Can you work these out from the model? Positions are in its coordinate system, mm. A direction names the side the tool comes from. Round coordinates to 2 decimals unless told otherwise and drop trailing zeros. Loops run counter-clockwise (first coordinate to the right, second up) from the corner with the lowest first, then second, coordinate; pieces in that order, holes last. Notation, with made-up numbers: M -37,-2 L 17,-2 A26 cw 17,27 Z; hole C 3,16.5 d6. An arc over 180 degrees is marked long. Answer as CSV lines item,"result".
from build123d import *

# Parameters (mm, degrees)
EXTRUDE_1_DEPTH     = 2
SKETCH_2_R          = 3.5
EXTRUDE_2_DEPTH     = 5.7
CUT_EXTRUDE_START   = -4.7
CUT_EXTRUDE_1_DEPTH = 4.7
SKETCH_5_R          = 1.05
CUT_EXTRUDE_2_DEPTH = 10
SKETCH_6_R          = 2
EXTRUDE_3_DEPTH     = 2
FILLET_1_R          = 2
SKETCH_7_R          = 1.05
CUT_EXTRUDE_3_DEPTH = 2
FILLET_2_R          = 0.4
CHAMFER_1_SIZE      = 2
CHAMFER_2_SIZE      = 0.4
SKETCH_8_R          = 3
SKETCH_8_R_2        = 2
CUT_EXTRUDE_5_DEPTH = 51.37135361
CHAMFER_3_SIZE      = 0.2


with BuildPart() as part:
    # 草图1 → 凸台-拉伸1 (new body)
    with BuildSketch(Plane(origin=(0, 0, 0), x_dir=(1, 0, 0), z_dir=(0, 1, 0))):
        Polygon((0.701628422, -0.113501573), (0.701628422, 23.886498427), (-2.298371578, 26.886498427), (-9.298371578, 26.886498427), (-9.298371578, 37.886498427), (24.701628422, 37.886498427), (32.701628422, 29.886498427), (32.701628422, -0.113501573), align=None)
    extrude(amount=EXTRUDE_1_DEPTH)

    # 草图2 → 凸台-拉伸2 (add)
    with BuildSketch(Plane.XZ):
        with Locations(Location((16.701628422, -17.136498427, 0), (0, 0, 270))):
            Circle(SKETCH_2_R)
        with BuildLine():
            ThreePointArc((15.171922568, -17.636498427), (16.701628422, -19.436498427), (18.231334277, -17.636498427))
            ThreePointArc((18.231334277, -17.636498427), (18.251628422, -17.386498427), (18.231334277, -17.136498427))
            ThreePointArc((18.231334277, -17.136498427), (18.251628422, -16.886498427), (18.231334277, -16.636498427))
            ThreePointArc((18.231334277, -16.636498427), (16.701628422, -14.836498427), (15.171922568, -16.636498427))
            ThreePointArc((15.171922568, -16.636498427), (15.151628422, -16.886498427), (15.171922568, -17.136498427))
            ThreePointArc((15.171922568, -17.136498427), (15.151628422, -17.386498427), (15.171922568, -17.636498427))
        make_face(mode=Mode.SUBTRACT)
    extrude(amount=EXTRUDE_2_DEPTH)

    # 草图3 → 切除-拉伸1 (cut)
    with BuildSketch(Plane.XZ.offset(CUT_EXTRUDE_START)):
        with BuildLine():
            ThreePointArc((15.171922568, -17.136498427), (15.151628422, -17.386498427), (15.171922568, -17.636498427))
            ThreePointArc((15.171922568, -17.636498427), (16.701628422, -19.436498427), (18.231334277, -17.636498427))
            ThreePointArc((18.231334277, -17.636498427), (18.251628422, -17.386498427), (18.231334277, -17.136498427))
            ThreePointArc((18.231334277, -17.136498427), (18.251628422, -16.886498427), (18.231334277, -16.636498427))
            ThreePointArc((18.231334277, -16.636498427), (16.701628422, -14.836498427), (15.171922568, -16.636498427))
            ThreePointArc((15.171922568, -16.636498427), (15.151628422, -16.886498427), (15.171922568, -17.136498427))
        make_face()
    extrude(amount=CUT_EXTRUDE_1_DEPTH, mode=Mode.SUBTRACT)

    # 草图5 → 切除-拉伸2 (cut)
    with BuildSketch(Plane.XZ):
        with Locations(Location((30.701628422, -28.886498427, 0), (0, 0, 270))):
            Circle(SKETCH_5_R)
        with Locations(Location((0.901628422, -27.086498427, 0), (0, 0, 270))):
            Circle(SKETCH_5_R)
    extrude(amount=-CUT_EXTRUDE_2_DEPTH, mode=Mode.SUBTRACT)

    # 草图6 → 凸台-拉伸3 (add)
    with BuildSketch(Plane(origin=(0, 0, 0), x_dir=(-1, 0, 0), z_dir=(0, -1, 0))):
        with Locations((-16.701628422, -0.113501573)):
            Circle(SKETCH_6_R)
    extrude(amount=-EXTRUDE_3_DEPTH)

    # 圆角1
    fillet_1_edges = [part.edges().sort_by_distance(p)[0] for p in [
        (18.701628422, 1, 0.113501573),
        (14.701628422, 1, 0.113501573),
    ]]
    fillet(fillet_1_edges, radius=FILLET_1_R)

    # 草图7 → 切除-拉伸3 (cut)
    with BuildSketch(Plane(origin=(0, 2, 0), x_dir=(1, 0, 0), z_dir=(0, 1, 0))):
        with Locations(Location((16.701628422, -0.113501573, 0), (0, 0, 270))):
            Circle(SKETCH_7_R)
    extrude(amount=-CUT_EXTRUDE_3_DEPTH, mode=Mode.SUBTRACT)

    # 圆角2
    fillet_2_edges = [part.edges().sort_by_distance(p)[0] for p in [
        (0.701628422, 1, 0.113501573),
        (0.701628422, 1, -23.886498427),
        (-2.298371578, 1, -26.886498427),
        (-9.298371578, 1, -26.886498427),
        (-9.298371578, 1, -37.886498427),
        (24.701628422, 1, -37.886498427),
        (32.701628422, 1, -29.886498427),
        (32.701628422, 1, 0.113501573),
    ]]
    fillet(fillet_2_edges, radius=FILLET_2_R)

    # 倒角1
    chamfer_1_edges = [part.edges().sort_by_distance(p)[0] for p in [
        (16.701628422, 0, -13.636498427),
    ]]
    chamfer(chamfer_1_edges, length=CHAMFER_1_SIZE)

    # 倒角2
    chamfer_2_edges = [part.edges().sort_by_distance(p)[0] for p in [
        (16.701628422, -5.7, -13.636498427),
    ]]
    chamfer(chamfer_2_edges, length=CHAMFER_2_SIZE)

    # 草图8 → 切除-拉伸5 (cut, through all)
    with BuildSketch(Plane.XZ):
        with Locations(Location((8.701628422, -7.886498427, 0), (0, 0, 270))):
            Circle(SKETCH_8_R)
        with Locations(Location((14.701628422, -29.886498427, 0), (0, 0, 270))):
            Circle(SKETCH_8_R_2)
    extrude(amount=-CUT_EXTRUDE_5_DEPTH, mode=Mode.SUBTRACT)

    # 倒角3
    chamfer_3_edges = [part.edges().sort_by_distance(p)[0] for p in [
        (26.23367923, 2, 0.113501573),
        (16.701628422, 2, 2.113501573),
        (19.165730038, 2, 0.381450765),
        (14.237526807, 2, 0.381450765),
        (16.701628422, 2, -0.936498427),
        (7.81878571, 2, -37.886498427),
        (28.701628422, 2, -33.886498427),
        (7.169577615, 2, 0.113501573),
        (32.701628422, 2, -15.003655715),
        (-9.298371578, 2, -32.386498427),
        (-5.68121429, 2, -26.886498427),
        (-0.798371578, 2, -25.386498427),
        (0.701628422, 2, -12.003655715),
        (-9.18121429, 2, -27.003655715),
        (-9.18121429, 2, -37.769341139),
        (0.81878571, 2, -0.003655715),
        (32.584471135, 2, -0.003655715),
        (32.671180235, 2, -29.873886375),
        (24.68901637, 2, -37.85605024),
        (0.671180235, 2, -23.873886375),
        (-2.31098363, 2, -26.85605024),
        (8.701628422, 2, -4.886498427),
        (14.701628422, 2, -27.886498427),
        (16.701628422, 2, -19.436498427),
        (18.251628422, 2, -17.386498427),
        (18.251628422, 2, -16.886498427),
        (16.701628422, 2, -14.836498427),
        (15.151628422, 2, -16.886498427),
        (15.151628422, 2, -17.386498427),
        (30.701628422, 2, -27.836498427),
        (0.901628422, 2, -26.036498427),
    ]]
    chamfer(chamfer_3_edges, length=CHAMFER_3_SIZE)


solid = part.part
Item 1: On a 3-axis mill with a long thin cutter (end or side, diameter ignored), from which of +Z, -Z, +X, -X, +Y, -Y can I reach the whole of each face in a straight line? I mean faces 1 (the face through (26, 1, 0.114)), 2 (the face through (7, 1, 0.114)), 3 (the face through (8, 1, -37.886)). Say none if no direction works.
Output:
face 1,"+Z, +X, +Y, -Y"
face 2,"+Z, -X, +Y, -Y"
face 3,"-Z, +X, -X, +Y, -Y"
Item 2: If we section it at D-D on z = -4: Write out the boundary of the cut face in (x, y), then the cut area to 3 significant figures.
Output:
outline,"M 0.7,0 L 32.7,0 L 32.7,1.8 L 32.5,2 L 0.9,2 L 0.7,1.8 Z"
area,"64.0 mm2"
Item 3: Will these pins go through, and if not, where does the flat tip stop? pin 1 (9.5 mm diameter, centred on x = 8.7, z = -7.89, fed in from -Y); pin 2 (0.5 mm diameter, centred on y = 0.5, z = -10, fed in from -X); pin 3 (2 mm diameter, centred on x = 27.5, y = 1, fed in from +Z).
Output:
pin 1,"stops at y = 0"
pin 2,"stops at x = 0.7"
pin 3,"stops at z = 0.11"
Item 4: If we section it at C-C on y = 0.5: State how many separate pieces and enclosed holes the cut face has, then the cut area to 3 significant figures.
Output:
separate pieces,"1"
enclosed holes,"6"
area,"1,240 mm2"
Item 5: We'd pull the mould along Z, two halves only. Please class faces 4 (the face through (-6, 1, -26.886)), 5 (the face through (16.664, -1.898, -19.436)), 6 (the face through (19.65, -3.63, -19.02)), 7 (the face through (0.702, 1, -12)): released by +Z, released by -Z, zero draft, split by the parting line, or undercut.
Output:
face 4,"released by +Z"
face 5,"undercut"
face 6,"split by the parting line"
face 7,"zero draft"
Item 6: If we section it at A-A on y = -2.75: Write out the boundary of the cut face in (x, z), then the cut area to 3 significant figures.
Output:
outline,"C 16.7,-17.14 d7; hole M 15.17,-17.64 A1.55 ccw long 18.23,-17.64 A1.55 ccw 18.23,-17.14 A1.55 ccw 18.23,-16.64 A1.55 ccw long 15.17,-16.64 A1.55 ccw 15.17,-17.14 A1.55 ccw Z"
area,"26.3 mm2"
Item 7: If I drill on line 1 along Y through (x, z) = (26, -5); line 2 along X through (y, z) = (0.25, -8); line 3 along X through (y, z) = (-2, -17), over which ranges is the centre line in solid material (lowest first)? Write a range as from..to.
Output:
line 1,"y = 0..2"
line 2,"x = 0.7..5.7, 11.7..32.7"
line 3,"x = 13.2..15.16, 18.25..20.2"
Item 8: If we section it at B-B on x = -3: Write out the boundary of the cut face in (y, z), then the cut area to 3 significant figures.
Output:
outline,"M 0,-37.89 L 1.8,-37.89 L 2,-37.69 L 2,-27.09 L 1.8,-26.89 L 0,-26.89 Z"
area,"22.0 mm2"
